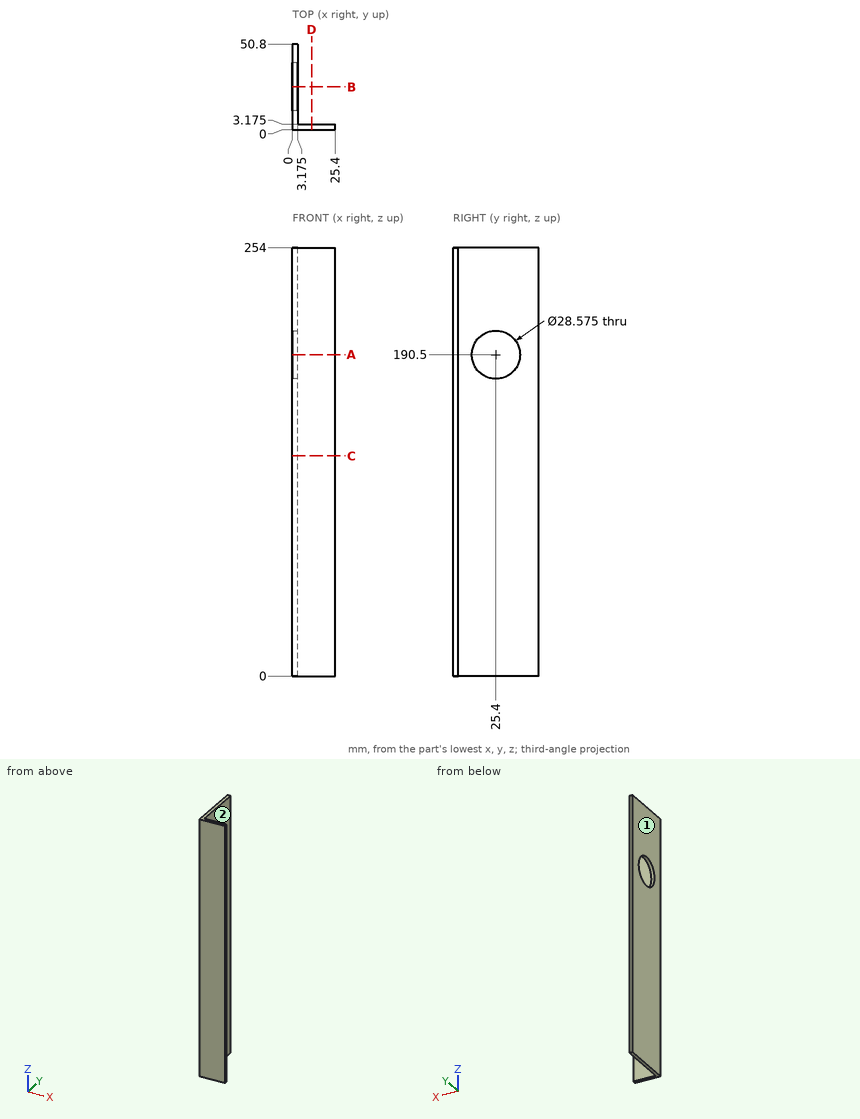
Drawing for the job (mm, zero at the part's lowest x, y, z). A direction names the side the tool comes from. Round coordinates to 2 decimals unless told otherwise and drop trailing zeros. Loops run counter-clockwise (first coordinate to the right, second up) from the corner with the lowest first, then second, coordinate; pieces in that order, holes last. Notation, with made-up numbers: (53.5, 76.5) -> (80.5, 76.5) arc R12 ccw to (80.5, 80.5) -> close; hole circle Ø5 at (-17.75, 1). An arc over 180 degrees is marked (long way). Answer as CSV lines item,"result". Start each with the question number.
1) Slice it at B-B (y = 25.4). List the corners of the cut face in (x, z) (1 decimal).
2) Pin check, flat tips, straight feed: P1, Ø5, axis at x = 16.5, z = 113.5, coming from the +Y side (3 decimals); P2, Ø2, axis at y = 34, z = 200.5, coming from the +X side; P3, Ø14.5, axis at y = 38.5, z = 136.5, coming from the +X side (3 decimals). Stop position of each tip, or through.
3) Slice it at C-C (z = 130.5). List the corners of the cut face in (x, y) (3 decimals), plus the area to 3 significant figures.
4) Probe line 1 along Y through (x, z) = (2.25, 190.5); line 2 along X through (y, z) = (32.5, 18.5) (3 decimals). List the from-to ranges inside material, lowest first.
5) Tool access for the marked faces 1 and 2: list every direction of +Z, -Z, +X, -X, +Y, -Y with a clear straight run to the whole face (end or side of a thin tool).
6) Slice it at A-A (z = 190.5). List the corners of the cut face in (x, y) (1 decimal), plus the area to 3 significant figures.
7) Slice it at D-D (x = 11.5). List the corners of the cut face in (y, z) (3 decimals).
Filled in:
1,outline,"(0, 0) -> (3.2, 0) -> (3.2, 176.2) -> (0, 176.2) -> close; (0, 204.8) -> (3.2, 204.8) -> (3.2, 254) -> (0, 254) -> close"
2,P1,"stops at y = 3.175"
2,P2,"passes through"
2,P3,"stops at x = 3.175"
3,outline,"(0, 0) -> (25.4, 0) -> (25.4, 3.175) -> (3.175, 3.175) -> (3.175, 50.8) -> (0, 50.8) -> close"
3,area,"232 mm2"
4,line 1,"y = 0 to 11.11, 39.69 to 50.8"
4,line 2,"x = 0 to 3.175"
5,face 1,"+Z, -Z, -X, +Y, -Y"
5,face 2,"+Z, -Z, +X, +Y"
6,outline,"(0, 0) -> (25.4, 0) -> (25.4, 3.2) -> (3.2, 3.2) -> (3.2, 11.1) -> (0, 11.1) -> close; (0, 39.7) -> (3.2, 39.7) -> (3.2, 50.8) -> (0, 50.8) -> close"
6,area,"141 mm2"
7,outline,"(0, 0) -> (3.175, 0) -> (3.175, 254) -> (0, 254) -> close"
